Answer from the drawing. Dimensions are ordinates in mm from the lowest x, y and z of the part. A direction names the side the tool comes from. Round coordinates to 2 decimals unless told otherwise and drop trailing zeros. Order: outer loops, then holes, each group sorted by start corner. A loop starts at its lowest first (then second) coordinate and runs counter-clockwise, first axis right, second up. Notation, with made-up numbers: (33.25, 82.5) -> (76.25, 82.5) arc R29 ccw to (76.25, 103.5) -> close; hole circle Ø5 at (18.25, -10.75). An arc over 180 degrees is marked (long way). Use a Markdown table: item, result. Add a question column.
1. Consider L1, parallel to X at y = 7.65, z = 14.5; L2, parallel to Y at x = 17.5, z = 16.75; L3, parallel to Y at x = 9.25, z = 7.5. Determine where each line is inside the solid, lowest interval first. Write a range as [from, to].
2. Section C-C, the plane y = 7.75 is taken. Give the vertices of the cut face in (x, z).
3. The mould has two halves that part along Z. Classify the marked faces 3, 4 and 5: +Z half, -Z half, draft (parallel to the pull), parting line (faces both ways), or undercut.
4. Section D-D, the plane y = 1.25 is taken. Give the vertices of the cut face in (x, z).
5. For the marked faces 1 and 2, determine the directions among +Z, -Z, +X, -X, +Y, -Y from which every point of the face is accessible in a straight line to the end or side of a thin tool.
6. Section A-A, the plane x = 14.5 is taken. Give the vertices of the cut face in (y, z), then the cut area to 3 significant figures.
7. Given pin 1 (2 mm diameter, centred on x = 11.5, y = 4.5, fed in from -Z); pin 2 (1 mm diameter, centred on x = 25, z = 11.5, fed in from +Y); pin 3 (2 mm diameter, centred on y = 6, z = 9.5, fed in from -X); pin 4 (5 mm diameter, centred on x = 14.5, z = 14.5, fed in from -Y), each flat-ended and moving along its own axis, determine where each tip first touches the part or whether it passes through.
8. Section B-B, the plane z = 14.5 is taken. Give the vertices of the cut face in (x, y), then the cut area to 3 significant figures.
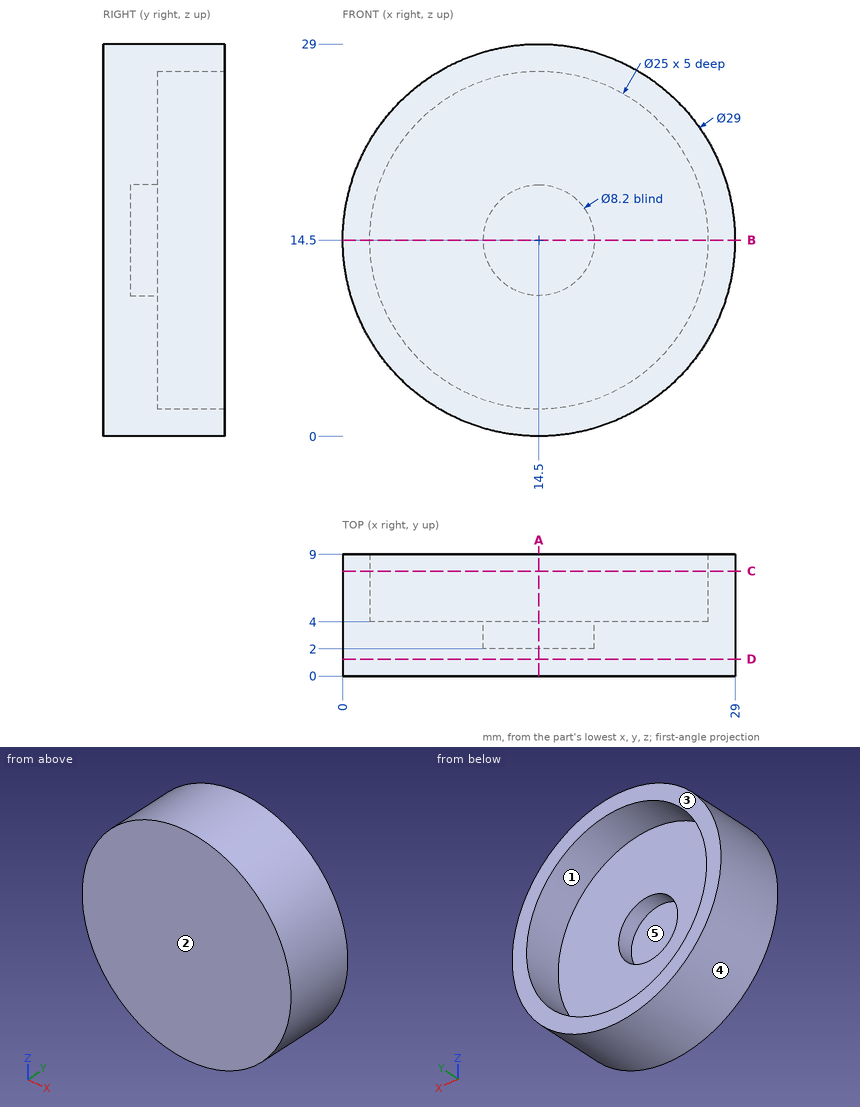
Verdict:
| question | item | result |
|---|---|---|
| 1 | L1 | x = [0, 2], [27, 29] |
| 1 | L2 | y = [0, 2] |
| 1 | L3 | y = [0, 4] |
| 2 | outline | circle Ø29 at (14.5, 14.5); hole circle Ø25 at (14.5, 14.5) |
| 3 | face 3 | draft |
| 3 | face 4 | parting line |
| 3 | face 5 | undercut |
| 4 | outline | circle Ø29 at (14.5, 14.5) |
| 5 | face 1 | +Y |
| 5 | face 2 | +Z, -Z, +X, -X, -Y |
| 6 | outline | (0, 0) -> (9, 0) -> (9, 2) -> (4, 2) -> (4, 10.4) -> (2, 10.4) -> (2, 18.6) -> (4, 18.6) -> (4, 27) -> (9, 27) -> (9, 29) -> (0, 29) -> close |
| 6 | area | 120 mm2 |
| 7 | pin 1 | stops at z = 0.14 |
| 7 | pin 2 | stops at y = 4 |
| 7 | pin 3 | stops at x = 0.56 |
| 7 | pin 4 | stops at y = 0 |
| 8 | outline | (0, 0) -> (29, 0) -> (29, 9) -> (27, 9) -> (27, 4) -> (18.6, 4) -> (18.6, 2) -> (10.4, 2) -> (10.4, 4) -> (2, 4) -> (2, 9) -> (0, 9) -> close |
| 8 | area | 120 mm2 |
